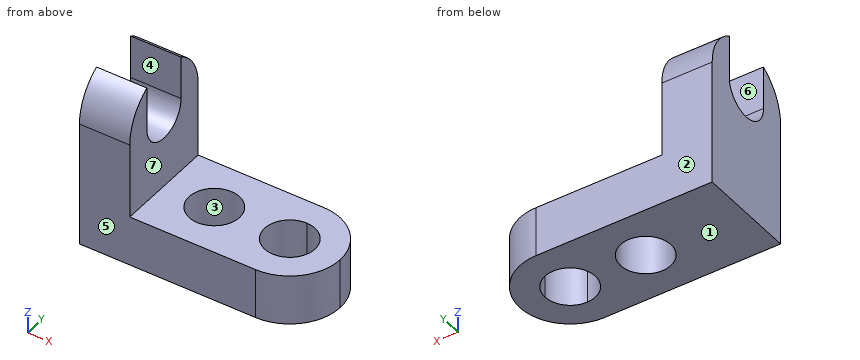
from build123d import *

# Parameters (mm, degrees)
F1_DEPTH = 25.4
F2_R     = 6.35
F3_DEPTH = 12.701
F5_DEPTH = 12.701


with BuildPart() as f1:
    # F0 (on Front) → F1 (new body)
    with BuildSketch(Plane.XZ):
        Polygon((-57.2872110233, 59.9430727009), (-69.9872110233, 59.9430727009), (-69.9872110233, 15.4930727009), (-12.8372110233, 15.4930727009), (-12.8372110233, 28.1930727009), (-57.2872110233, 28.1930727009), align=None)
    extrude(amount=F1_DEPTH)

    # F2 (on face) → F3 (cut, through all)
    with BuildSketch(Plane.XY.offset(28.1930727009)):
        with BuildLine():
            ThreePointArc((-12.8372110233, -12.7000000115), (-16.5569549063, -21.6802561251), (-25.5372110233, -25.4))
            Line((-25.5372110233, -25.4), (-12.8372110233, -25.4))
            Line((-12.8372110233, -25.4), (-12.8372110233, -12.7000000115))
        make_face()
        with BuildLine():
            Line((-12.8372110233, 0), (-25.5372110233, 0))
            ThreePointArc((-25.5372110233, 0), (-16.5569548981, -3.719743883), (-12.8372110233, -12.7000000115))
            Line((-12.8372110233, -12.7000000115), (-12.8372110233, 0))
        make_face()
        with BuildLine():
            ThreePointArc((-25.5372110233, -19.05), (-21.0470829627, -17.1901280605), (-19.1872110233, -12.7))
            ThreePointArc((-19.1872110233, -12.7), (-21.0470829627, -8.2098719395), (-25.5372110233, -6.35))
            ThreePointArc((-25.5372110233, -6.35), (-31.8872110233, -12.7), (-25.5372110233, -19.05))
        make_face()
        with Locations((-44.5872110233, -12.7)):
            Circle(F2_R)
    extrude(amount=-F3_DEPTH, mode=Mode.SUBTRACT)

    # F4 (on face) → F5 (cut, through all)
    with BuildSketch(Plane.YZ.offset(-57.2872110233)):
        with BuildLine():
            Line((-25.4, 59.9430727009), (-25.4, 47.2430727009))
            ThreePointArc((-25.4, 47.2430727009), (-23.6985226281, 53.5930727009), (-19.05, 58.2415953289))
            Line((-19.05, 58.2415953289), (-19.05, 59.9430727009))
            Line((-19.05, 59.9430727009), (-25.4, 59.9430727009))
        make_face()
        with BuildLine():
            ThreePointArc((-6.35, 58.2415953289), (-1.7014773719, 53.5930727009), (0, 47.2430727009))
            Line((0, 47.2430727009), (0, 59.9430727009))
            Line((0, 59.9430727009), (-6.35, 59.9430727009))
            Line((-6.35, 59.9430727009), (-6.35, 58.2415953289))
        make_face()
        with BuildLine():
            ThreePointArc((-12.7, 59.9430727009), (-9.4129981272, 59.5103306947), (-6.35, 58.2415953289))
            Line((-6.35, 58.2415953289), (-6.35, 59.9430727009))
            Line((-6.35, 59.9430727009), (-12.7, 59.9430727009))
        make_face()
        with BuildLine():
            Line((-19.05, 59.9430727009), (-19.05, 58.2415953289))
            ThreePointArc((-19.05, 58.2415953289), (-15.9870018728, 59.5103306947), (-12.7, 59.9430727009))
            Line((-12.7, 59.9430727009), (-19.05, 59.9430727009))
        make_face()
        with BuildLine():
            Line((-12.7, 47.2430727009), (-6.35, 47.2430727009))
            ThreePointArc((-6.35, 47.2430727009), (-12.7, 53.5930727009), (-19.05, 47.2430727009))
            Line((-19.05, 47.2430727009), (-12.7, 47.2430727009))
        make_face()
        with BuildLine():
            ThreePointArc((-19.05, 47.2430727009), (-12.7, 40.8930727009), (-6.35, 47.2430727009))
            Line((-6.35, 47.2430727009), (-12.7, 47.2430727009))
            Line((-12.7, 47.2430727009), (-19.05, 47.2430727009))
        make_face()
        with BuildLine():
            ThreePointArc((-19.05, 47.2430727009), (-12.7, 53.5930727009), (-6.35, 47.2430727009))
            Line((-6.35, 47.2430727009), (-6.35, 58.2415953289))
            ThreePointArc((-6.35, 58.2415953289), (-9.4129981272, 59.5103306947), (-12.7, 59.9430727009))
            ThreePointArc((-12.7, 59.9430727009), (-15.9870018728, 59.5103306947), (-19.05, 58.2415953289))
            Line((-19.05, 58.2415953289), (-19.05, 47.2430727009))
        make_face()
    extrude(amount=-F5_DEPTH, mode=Mode.SUBTRACT)


solid = f1.part
Build history of the part. All positions in model axes, mm. Face numbers are marked on the shaded views. A direction names the side the tool comes from. Coordinates: 2 decimals unless noted, no trailing zeros. Order: outer loops, then holes, each group sorted by start corner. A loop starts at its lowest first (then second) coordinate and runs counter-clockwise, first axis right, second up. Notation, with made-up numbers: (23, 57) - (27, 57) arc R6 ccw to (27, 67) - close; hole circle Ø10 at (9, 24). An arc over 180 degrees is marked (long way). Write item = value, one per line. Start each with the question number.
1) Two-plate mould, pull along Y, no slides. Class the marked faces 1, 2, 3 and 4: pulls with the +Y half, pulls with the -Y half, needs draft (parallel to the pull), parting line crosses it, or undercut.
2) Saw through at D-D on x = -40. Write the cut outline in (y, z).
3) Saw through at B-B on y = -11.5. Write the cut outline in (x, z).
4) Saw through at C-C on z = 21. Write the cut outline in (x, y).
5) 3-axis set-ups, long thin cutter, end or side, ignore diameter. For the marked faces 5, 6 and 7: which of +Z, -Z, +X, -X, +Y, -Y reach the whole face in a straight line?
6) Wall check: line 1 along X through (y, z) = (-18.5, 26); line 2 along Z through (x, y) = (-36.5, -3.75); line 3 along X through (y, z) = (-10, 32). Give the ranges that are in metal, low to high. Write a range as from..to.
7) Flat gauge pins, fed straight in: pin 1 Ø1 at (y, z) = (-18.5, 39.5) entering from +X; pin 2 Ø1 at (x, y) = (-34.5, -7) entering from +Z; pin 3 Ø4 at (y, z) = (-3, 25.5) entering from +X; pin 4 Ø12 at (x, z) = (-62, 51) entering from -Y. Where does each tip first touch, or does it go through?
8) Saw through at A-A on x = -21. Write the cut outline in (y, z), then the cut area to 3 significant figures.
From the geometry:
q1.face_1 = needs draft
q1.face_2 = pulls with the +Y half
q1.face_3 = undercut
q1.face_4 = undercut
q2.outline = (-25.4, 15.49) - (-17.09, 15.49) - (-17.09, 28.19) - (-25.4, 28.19) - close; (-8.31, 15.49) - (0, 15.49) - (0, 28.19) - (-8.31, 28.19) - close
q3.outline = (-69.99, 15.49) - (-50.82, 15.49) - (-50.82, 28.19) - (-57.29, 28.19) - (-57.29, 41.01) - (-69.99, 41.01) - close; (-38.35, 15.49) - (-31.77, 15.49) - (-31.77, 28.19) - (-38.35, 28.19) - close; (-19.3, 15.49) - (-12.89, 15.49) - (-12.89, 28.19) - (-19.3, 28.19) - close
q4.outline = (-69.99, -25.4) - (-25.54, -25.4) arc R12.7 ccw to (-25.54, 0) - (-69.99, 0) - close; hole circle Ø12.7 at (-44.59, -12.7); hole circle Ø12.7 at (-25.54, -12.7)
q5.face_5 = +Z, -Z, +X, -X, -Y
q5.face_6 = +Z, +X, -X
q5.face_7 = +Z, +X, +Y, -Y
q6.line_1 = -69.99..-47.17, -42..-28.12, -22.95..-14.24
q6.line_2 = 15.49..28.19
q6.line_3 = -69.99..-57.29
q7.pin_1 = -57.29
q7.pin_2 = 28.19
q7.pin_3 = -15.44
q7.pin_4 = -25.4
q8.outline = (-24.56, 15.49) - (-17.14, 15.49) - (-17.14, 28.19) - (-24.56, 28.19) - close; (-8.26, 15.49) - (-0.84, 15.49) - (-0.84, 28.19) - (-8.26, 28.19) - close
q8.area = 188 mm^2
